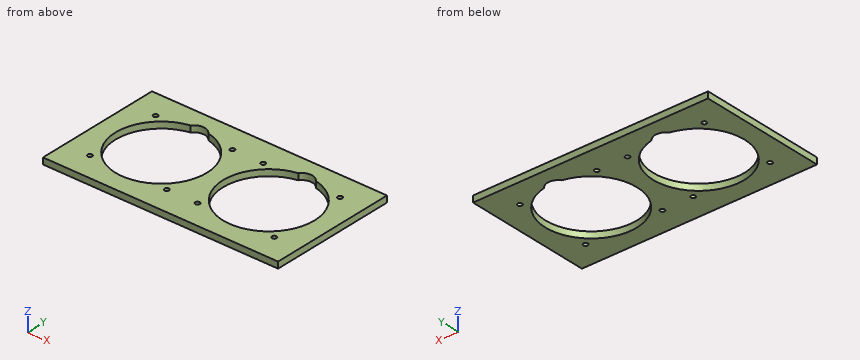
```python
from build123d import *

# Parameters (mm, degrees)
F0_W     = 130
F0_H     = 70.5
F1_DEPTH = 3.5
F2_D     = 2.5


# Not quite as in the source:
# - a feature names something its author has since deleted; it is built from what else it names


with BuildPart() as f1:
    # F0 (on Top) → F1 (new body)
    with BuildSketch(Plane.XY):
        Rectangle(F0_W, F0_H)
        with BuildLine():
            ThreePointArc((-24.8978610289, 24.7794117647), (-29.75, -25.25), (-34.6021389711, 24.7794117647))
            ThreePointArc((-34.6021389711, 24.7794117647), (-29.75, 27.25), (-24.8978610289, 24.7794117647))
        make_face(mode=Mode.SUBTRACT)
        with BuildLine():
            ThreePointArc((34.6021389711, 24.7794117647), (29.75, -25.25), (24.8978610289, 24.7794117647))
            ThreePointArc((24.8978610289, 24.7794117647), (29.75, 27.25), (34.6021389711, 24.7794117647))
        make_face(mode=Mode.SUBTRACT)
    extrude(amount=F1_DEPTH)

    # F2 (through all)
    with Locations(Plane(origin=(0, 0, 0), x_dir=(1, 0, 0), z_dir=(0, 0, -1))):
        with Locations((-51, -21.25), (-51, 21.25), (-8.5, 21.25), (-8.5, -21.25), (8.5, -21.25), (8.5, 21.25), (51, 21.25), (51, -21.25)):
            Hole(F2_D / 2)


solid = f1.part
```
Read the model definition and answer for the solid it produces. Units are mm, in the model's axes. Coordinates: 2 decimals unless noted, no trailing zeros. Write each loop counter-clockwise with the first axis right and the second up, starting at its lowest first coordinate (ties: lowest second). Pieces come first, ordered by that corner, then holes. Notation, with made-up numbers: (89, -3) -> (108, -3) arc R27 cw to (108, 26) -> close; hole circle Ø11 at (-31, 41.5). An arc over 180 degrees is marked (long way). Write item = value, one per line.
(1) Section C-C on z = 2.45 is taken. Count the separate pieces of the cut face and the enclosed holes in it, plus the area to 3 significant figures.
From the geometry:
separate_pieces = 1
enclosed_holes = 10
area = 5,090 mm2
(2) Given pin 1 Ø3 at (x, y) = (-51, -21.25) entering from +Z, flat-ended and moving along its own axis, determine where the tip first touches the part or whether it passes through.
From the geometry:
pin_1 = 3.5
(3) Section A-A on x = 29.75 is taken. Write down the section's boundary in (y, z).
From the geometry:
outline = (-35.25, 0) -> (-25.25, 0) -> (-25.25, 3.5) -> (-35.25, 3.5) -> close; (27.25, 0) -> (35.25, 0) -> (35.25, 3.5) -> (27.25, 3.5) -> close
(4) Straight lines are drawn through the part: L1, parallel to X at y = 0, z = 2.6; L2, parallel to X at y = 26.5, z = 2.8; L3, parallel to Y at x = -51, z = 1.5. For each, find the intervals that lie inside material, in ascending order. Write a range as from..to.
From the geometry:
L1 = -65..-55, -4.5..4.5, 55..65
L2 = -65..-32.65, -26.85..26.85, 32.65..65
L3 = -35.25..-22.5, -20..-13.64, 13.64..20, 22.5..35.25
(5) Section B-B on y = 21.25 is taken. Write down the section's boundary in (x, z).
From the geometry:
outline = (-65, 0) -> (-52.25, 0) -> (-52.25, 3.5) -> (-65, 3.5) -> close; (-49.75, 0) -> (-43.39, 0) -> (-43.39, 3.5) -> (-49.75, 3.5) -> close; (-16.11, 0) -> (-9.75, 0) -> (-9.75, 3.5) -> (-16.11, 3.5) -> close; (-7.25, 0) -> (7.25, 0) -> (7.25, 3.5) -> (-7.25, 3.5) -> close; (9.75, 0) -> (16.11, 0) -> (16.11, 3.5) -> (9.75, 3.5) -> close; (43.39, 0) -> (49.75, 0) -> (49.75, 3.5) -> (43.39, 3.5) -> close; (52.25, 0) -> (65, 0) -> (65, 3.5) -> (52.25, 3.5) -> close
(6) Section D-D on x = -51 is taken. Write down the section's boundary in (y, z), plus the area to 3 significant figures.
From the geometry:
outline = (-35.25, 0) -> (-22.5, 0) -> (-22.5, 3.5) -> (-35.25, 3.5) -> close; (-20, 0) -> (-13.64, 0) -> (-13.64, 3.5) -> (-20, 3.5) -> close; (13.64, 0) -> (20, 0) -> (20, 3.5) -> (13.64, 3.5) -> close; (22.5, 0) -> (35.25, 0) -> (35.25, 3.5) -> (22.5, 3.5) -> close
area = 134 mm2
